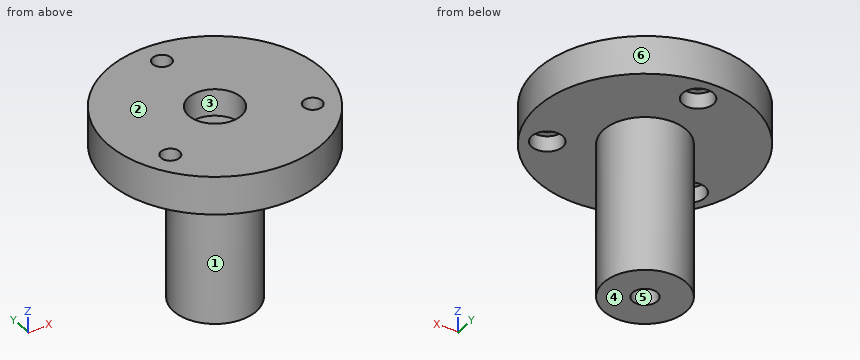
```python
from build123d import *

# Parameters (mm, degrees)
SKETCH_1_R               = 10.4
EXTRUDE_1_DEPTH          = 3.7
SKETCH_2_R               = 0.9
CUT_EXTRUDE_1_DEPTH      = 16.166080575
SKETCH_2_3_R             = 1.5
CUT_EXTRUDE_2_DEPTH      = 1.5
PATTERN_CIRCULAR_1_COUNT = 3
SKETCH_3_R               = 1.2
CUT_EXTRUDE_3_DEPTH      = 16.166080575
SKETCH_4_R               = 2.55
CUT_EXTRUDE_4_DEPTH      = 2.6
EXTRUDE_START            = 15
SKETCH_5_R               = 4
SKETCH_5_R_2             = 1.2
EXTRUDE_2_DEPTH          = 15


with BuildPart() as part:
    # Sketch 1 → Extrude 1 (new body)
    with BuildSketch(Plane.XY):
        Circle(SKETCH_1_R)
    extrude(amount=EXTRUDE_1_DEPTH)

    # Sketch 2 → Cut-Extrude 1 (cut, through all)
    with BuildSketch(Plane(origin=(0, 0, 0), x_dir=(-1, 0, 0), z_dir=(0, 0, -1))):
        with Locations((0, 8)):
            Circle(SKETCH_2_R)
    cut_extrude_1 = extrude(amount=-CUT_EXTRUDE_1_DEPTH, mode=Mode.SUBTRACT)

    # Sketch 2_3 → Cut-Extrude 2 (cut)
    with BuildSketch(Plane(origin=(0, 0, 0), x_dir=(-1, 0, 0), z_dir=(0, 0, -1))):
        with Locations((0, 8)):
            Circle(SKETCH_2_3_R)
    cut_extrude_2 = extrude(amount=-CUT_EXTRUDE_2_DEPTH, mode=Mode.SUBTRACT)

    # Pattern Circular 1: Cut-Extrude 1, Cut-Extrude 2 ×3 about axis
    pattern_circular_1_axis = Axis((0, 0, 0), (0, 0, 1))
    add([cut_extrude_1.rotate(pattern_circular_1_axis, i * 360 / PATTERN_CIRCULAR_1_COUNT) for i in range(1, PATTERN_CIRCULAR_1_COUNT)], mode=Mode.SUBTRACT)
    add([cut_extrude_2.rotate(pattern_circular_1_axis, i * 360 / PATTERN_CIRCULAR_1_COUNT) for i in range(1, PATTERN_CIRCULAR_1_COUNT)], mode=Mode.SUBTRACT)

    # Sketch 3 → Cut-Extrude 3 (cut, through all)
    with BuildSketch(Plane(origin=(0, 0, 0), x_dir=(-1, 0, 0), z_dir=(0, 0, -1))):
        Circle(SKETCH_3_R)
    extrude(amount=-CUT_EXTRUDE_3_DEPTH, mode=Mode.SUBTRACT)

    # Sketch 4 → Cut-Extrude 4 (cut)
    with BuildSketch(Plane.XY.offset(3.7)):
        Circle(SKETCH_4_R)
    extrude(amount=-CUT_EXTRUDE_4_DEPTH, mode=Mode.SUBTRACT)

    # Sketch 5 → Extrude 2 (add)
    with BuildSketch(Plane(origin=(0, 0, 0), x_dir=(-1, 0, 0), z_dir=(0, 0, -1)).offset(EXTRUDE_START)):
        Circle(SKETCH_5_R)
        Circle(SKETCH_5_R_2, mode=Mode.SUBTRACT)
    extrude(amount=-EXTRUDE_2_DEPTH)


solid = part.part
```
The listing builds one solid part. Answer for the finished solid, in the listing's coordinates (mm). Face numbers are marked on the shaded views. A direction names the side the tool comes from. Give positions to 0.01 mm unless a question says otherwise; leave off trailing zeros. Write each loop counter-clockwise with the first axis right and the second up, starting at its lowest first coordinate (ties: lowest second). Pieces come first, ordered by that corner, then holes. Notation, with made-up numbers: (9, -35.5) -> (54, -35.5) arc R25 ccw to (54, -7.5) -> close; hole circle Ø3 at (69.25, 8.5). An arc over 180 degrees is marked (long way). Write item = value, one per line. Start each with the question number.
1) Which of the six approach directions +Z, -Z, +X, -X, +Y, -Y give full straight-line access (tool end or side, diameter ignored) to the marked faces 1, 2 and 3?
2) The part is cut by section B-B, the plane x = 0. Determine the outline of the cut face in (y, z), and give its area (3 significant figures).
3) The part is cut by section A-A, the plane y = 0. Determine the outline of the cut face in (x, z), and give its area (3 significant figures).
4) The part is cut by section D-D, the plane z = -5. Determine the outline of the cut face in (x, y).
5) Straight lines are drawn through the part: line 1 along Y through (x, z) = (0, 2.45); line 2 along Y through (x, z) = (0, 0.9); line 3 along Z through (x, y) = (7.75, 2.5). For each, find the intervals that lie inside material, in ascending order.
6) Each of these flat-tipped pins is pushed along its axis until it touches: pin 1 (1.5 mm diameter, centred on x = 2, z = -7, fed in from -Y); pin 2 (3.5 mm diameter, centred on x = -7.5, y = -3.5, fed in from -Z); pin 3 (2.5 mm diameter, centred on x = 1, y = 0.5, fed in from +Z). Where does it stop, or does it pass through?
7) The part is cut by section C-C, the plane x = -7.25. Determine the outline of the cut face in (y, z), and give its area (3 significant figures).
8) Determine the mould class of the marked faces 4, 5 and 6 for opening direction Y: +Y half, -Y half, draft (parallel to the pull), parting line (faces both ways), or undercut.
Solutions:
q1.face_1 = -Z
q1.face_2 = +Z, +X, -X, +Y, -Y
q1.face_3 = +Z
q2.outline = (-10.4, 0) -> (-4, 0) -> (-4, -15) -> (-1.2, -15) -> (-1.2, 1.1) -> (-2.55, 1.1) -> (-2.55, 3.7) -> (-10.4, 3.7) -> close; (1.2, -15) -> (4, -15) -> (4, 0) -> (6.5, 0) -> (6.5, 1.5) -> (7.1, 1.5) -> (7.1, 3.7) -> (2.55, 3.7) -> (2.55, 1.1) -> (1.2, 1.1) -> close; (8.9, 1.5) -> (9.5, 1.5) -> (9.5, 0) -> (10.4, 0) -> (10.4, 3.7) -> (8.9, 3.7) -> close
q2.area = 137 mm²
q3.outline = (-10.4, 0) -> (-4, 0) -> (-4, -15) -> (-1.2, -15) -> (-1.2, 1.1) -> (-2.55, 1.1) -> (-2.55, 3.7) -> (-10.4, 3.7) -> close; (1.2, -15) -> (4, -15) -> (4, 0) -> (10.4, 0) -> (10.4, 3.7) -> (2.55, 3.7) -> (2.55, 1.1) -> (1.2, 1.1) -> close
q3.area = 145 mm²
q4.outline = circle Ø8 at (0, 0); hole circle Ø2.4 at (0, 0)
q5.line_1 = -10.4 to -2.55, 2.55 to 7.1, 8.9 to 10.4
q5.line_2 = -10.4 to -1.2, 1.2 to 6.5, 9.5 to 10.4
q5.line_3 = 0 to 3.7
q6.pin_1 = -3.8
q6.pin_2 = 0
q6.pin_3 = 1.1
q7.outline = (-7.46, 0) -> (-5.47, 0) -> (-5.47, 1.5) -> (-4.84, 1.5) -> (-4.84, 3.7) -> (-7.46, 3.7) -> close; (-3.16, 1.5) -> (-2.53, 1.5) -> (-2.53, 0) -> (7.46, 0) -> (7.46, 3.7) -> (-3.16, 3.7) -> close
q7.area = 47.1 mm²
q8.face_4 = draft
q8.face_5 = undercut
q8.face_6 = parting line
